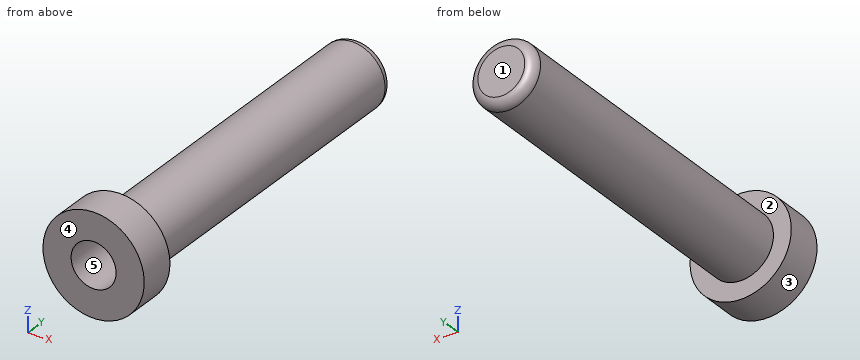
from build123d import *

# Parameters (mm, degrees)
SKETCH1_R           = 2.7
BOSS_EXTRUDE1_DEPTH = 2
SKETCH3_R           = 0.95
CUT_EXTRUDE2_DEPTH  = 9.5
SKETCH2_R           = 1.75
BOSS_EXTRUDE2_DEPTH = 18.6
SKETCH7_R           = 1.2
CUT_EXTRUDE4_DEPTH  = 2.8
FILLET2_R           = 0.5
SKETCH8_R           = 0.85
CUT_EXTRUDE5_DEPTH  = 10.5


with BuildPart() as part:
    # Sketch1 → Boss-Extrude1 (new body)
    with BuildSketch(Plane(origin=(0, 0, 0), x_dir=(1, 0, 0), z_dir=(0, 1, 0))):
        with Locations(Location((0, 0, 0), (0, 0, 270))):
            Circle(SKETCH1_R)
    extrude(amount=BOSS_EXTRUDE1_DEPTH)

    # Sketch3 → Cut-Extrude2 (cut)
    with BuildSketch(Plane.XZ):
        with Locations(Location((0, 0, 0), (0, 0, 270))):
            Circle(SKETCH3_R)
    extrude(amount=-CUT_EXTRUDE2_DEPTH, mode=Mode.SUBTRACT)

    # Sketch2 → Boss-Extrude2 (add)
    with BuildSketch(Plane(origin=(0, 2, 0), x_dir=(1, 0, 0), z_dir=(0, 1, 0))):
        with Locations(Location((0, 0, 0), (0, 0, 270))):
            Circle(SKETCH2_R)
    extrude(amount=BOSS_EXTRUDE2_DEPTH)

    # Sketch7 → Cut-Extrude4 (cut)
    with BuildSketch(Plane.XZ):
        with Locations(Location((0, 0, 0), (0, 0, 270))):
            Circle(SKETCH7_R)
    extrude(amount=-CUT_EXTRUDE4_DEPTH, mode=Mode.SUBTRACT)

    # Fillet2
    fillet2_edges = [part.edges().sort_by_distance(p)[0] for p in [
        (0, 20.6, -1.75),
    ]]
    fillet(fillet2_edges, radius=FILLET2_R)

    # Sketch8 → Cut-Extrude5 (cut)
    with BuildSketch(Plane.XZ):
        with Locations(Location((0, 0, 0), (0, 0, 270))):
            Circle(SKETCH8_R)
    extrude(amount=-CUT_EXTRUDE5_DEPTH, mode=Mode.SUBTRACT)


solid = part.part
Here's how the part is built. I have some questions about the finished solid (model axes, mm). Face numbers are marked on the shaded views. A direction names the side the tool comes from. Coordinates: 2 decimals unless noted, no trailing zeros. Write each loop counter-clockwise with the first axis right and the second up, starting at its lowest first coordinate (ties: lowest second). Pieces come first, ordered by that corner, then holes.
Item 1: Will these pins go through, and if not, where does the flat tip stop? pin 1 (1.9 mm diameter, centred on x = 0, z = 0, fed in from -Y); pin 2 (2 mm diameter, centred on x = 1.5, z = -2, fed in from +Y); pin 3 (2.5 mm diameter, centred on x = -0.5, z = 0, fed in from -Y); pin 4 (2 mm diameter, centred on x = -1, y = 15.5, fed in from +Z).
Item 2: On a 3-axis mill with a long thin cutter (end or side, diameter ignored), from which of +Z, -Z, +X, -X, +Y, -Y can I reach the whole of each face in a straight line? I mean the marked faces 1 and 2. Say none if no direction works.
Item 3: I want a section at C-C on y = 9.25. Write out the boundary of the cut face in (x, z), and give its area (3 significant figures).
Item 4: I want a section at A-A on z = 0. Write out the boundary of the cut face in (x, y).
Item 5: If we mould it in two halves opening along Z, with no side actions, what happens to the marked faces 3, 4 and 5? For each: +Z half, -Z half, draft (parallel to the pull), parting line (faces both ways), or undercut.
Item 6: If I drill on line 1 (X direction, y = 5.75, z = 0); line 2 (X direction, y = 0.9, z = 0); line 3 (Y direction, x = 0.4, z = -0.05), over which ranges is the centre line in solid material (lowest first)?
Item 7: I want a section at B-B on x = 0. Write out the boundary of the cut face in (y, z), and give its area (3 significant figures).
Item 8: I want a section at D-D on y = 17.25. Write out the boundary of the cut face in (x, z), and give its area (3 significant figures).
Findings below:
1. pin 1: stops at y = 2.8
1. pin 2: stops at y = 20.53
1. pin 3: stops at y = 0
1. pin 4: stops at z = 1.75
2. face 1: +Z, -Z, +X, -X, +Y
2. face 2: +Y
3. outline: circle Ø3.5 at (0, 0); hole circle Ø1.7 at (0, 0)
3. area: 7.35 mm2
4. outline: (-2.7, 0) - (-1.2, 0) - (-1.2, 2.8) - (-0.85, 2.8) - (-0.85, 10.5) - (0.85, 10.5) - (0.85, 2.8) - (1.2, 2.8) - (1.2, 0) - (2.7, 0) - (2.7, 2) - (1.75, 2) - (1.75, 20.1) arc R0.5 ccw to (1.25, 20.6) - (-1.25, 20.6) arc R0.5 ccw to (-1.75, 20.1) - (-1.75, 2) - (-2.7, 2) - close
5. face 3: parting line
5. face 4: draft
5. face 5: undercut
6. line 1: x = -1.75 to -0.85, 0.85 to 1.75
6. line 2: x = -2.7 to -1.2, 1.2 to 2.7
6. line 3: y = 10.5 to 20.6
7. outline: (0, -2.7) - (2, -2.7) - (2, -1.75) - (20.1, -1.75) arc R0.5 ccw to (20.6, -1.25) - (20.6, 1.25) arc R0.5 ccw to (20.1, 1.75) - (2, 1.75) - (2, 2.7) - (0, 2.7) - (0, 1.2) - (2.8, 1.2) - (2.8, 0.85) - (10.5, 0.85) - (10.5, -0.85) - (2.8, -0.85) - (2.8, -1.2) - (0, -1.2) - close
7. area: 56.0 mm2
8. outline: circle Ø3.5 at (0, 0)
8. area: 9.62 mm2
